from build123d import *

# Parameters (mm, degrees)
SKETCH2_W           = 54.8
SKETCH2_H           = 9.08
BOSS_EXTRUDE1_DEPTH = 6.49
SKETCH3_W           = 50
SKETCH3_H           = 6.43
CUT_EXTRUDE1_DEPTH  = 57.521498565
BOSS_EXTRUDE2_DEPTH = 6.49


with BuildPart() as part:
    # Sketch2 → Boss-Extrude1 (new body)
    with BuildSketch(Plane.XZ):
        with Locations((13.46, 33.97)):
            Rectangle(SKETCH2_W, SKETCH2_H)
    extrude(amount=BOSS_EXTRUDE1_DEPTH)

    # Sketch3 → Cut-Extrude1 (cut, through all)
    with BuildSketch(Plane(origin=(0, 0, 0), x_dir=(1, 0, 0), z_dir=(0, 1, 0))):
        with Locations((13.46, -32.645)):
            Rectangle(SKETCH3_W, SKETCH3_H)
    extrude(amount=-CUT_EXTRUDE1_DEPTH, mode=Mode.SUBTRACT)

    # Sketch4 → Boss-Extrude2 (add, through all)
    with BuildSketch(Plane(origin=(0, 0, 0), x_dir=(1, 0, 0), z_dir=(0, 1, 0))):
        with BuildLine():
            Line((38.46, -29.43), (37.86, -29.43))
            ThreePointArc((37.86, -29.43), (37.36, -30.68), (37.86, -31.93))
            Line((37.86, -31.93), (38.46, -31.93))
            Line((38.46, -31.93), (38.46, -29.43))
        make_face()
        with BuildLine():
            Line((-10.94, -31.93), (-11.54, -31.93))
            Line((-11.54, -31.93), (-11.54, -29.43))
            Line((-11.54, -29.43), (-10.94, -29.43))
            ThreePointArc((-10.94, -29.43), (-10.44, -30.68), (-10.94, -31.93))
        make_face()
    extrude(amount=-BOSS_EXTRUDE2_DEPTH)


solid = part.part
The model under review builds one solid part; all positions refer to its coordinate system, in mm. A direction names the side the tool comes from. Give positions to 0.01 mm unless a question says otherwise; leave off trailing zeros. Write each loop counter-clockwise with the first axis right and the second up, starting at its lowest first coordinate (ties: lowest second). Pieces come first, ordered by that corner, then holes. Notation, with made-up numbers: M 87.25,53 L 106.25,53 A17 cw 106.25,77 Z; hole C 33,44 d6. An arc over 180 degrees is marked long. One line per question, with ' | ' between items. Start each with the question number.
Item 1: For pin 1 (1.5 mm diameter, centred on x = -3.5, z = 34, fed in from -Y); pin 2 (1.9 mm diameter, centred on x = 18, y = -2, fed in from -Z), all flat-tipped, find the tip position at first contact; note any pin that passes through.
Item 2: Draft analysis for pull direction X (two halves, no side actions). For faces 3 (the flat face through (-13.94, -3, 34)), 4 (the flat face through (13, -6.49, 37)), 5 (the flat face through (38.46, -3, 34)), state which applies: released by +X, released by -X, zero draft, split by the parting line, or undercut.
Item 3: We need section B-B on y = -5.5. Write out the cut boundary in (x, z) (1 decimal), plus the area to 3 significant figures.
Item 4: We need section C-C on z = 31. Write out the cut boundary in (x, y).
Item 5: We need section A-A on z = 34.75. Write out the cut boundary in (x, y).
Item 6: Wall thickness on line 1 (X direction, y = -4.5, z = 32); line 2 (Z direction, x = 29.5, y = -5); line 3 (Z direction, x = -11, y = -5.25): over which ranges is each line inside the solid? List them lowest first. Write a range as from..to.
Item 7: For faces 1 (the flat face through (-12, -3, 29.43)), 2 (the flat face through (-11.54, -3, 34)), list the 3-axis set-ups (+Z, -Z, +X, -X, +Y, -Y) from which the entire face can be reached by the end or side of a thin tool; tool diameter is ignored.
Item 8: We need section D-D on x = 29. Write out the cut boundary in (y, z).
Results found:
1) pin 1: passes through | pin 2: stops at z = 35.86
2) face 3: released by -X | face 4: zero draft | face 5: undercut
3) outline: M -13.9,29.4 L -10.9,29.4 A1.8 ccw -10.9,31.9 L -11.5,31.9 L -11.5,35.9 L 38.5,35.9 L 38.5,31.9 L 37.9,31.9 A1.8 ccw 37.9,29.4 L 40.9,29.4 L 40.9,38.5 L -13.9,38.5 Z | area: 181 mm2
4) outline: M -13.94,-6.49 L -10.47,-6.49 L -10.47,0 L -13.94,0 Z; M 37.39,-6.49 L 40.86,-6.49 L 40.86,0 L 37.39,0 Z
5) outline: M -13.94,-6.49 L -11.54,-6.49 L -11.54,0 L -13.94,0 Z; M 38.46,-6.49 L 40.86,-6.49 L 40.86,0 L 38.46,0 Z
6) line 1: x = -13.94..-11.54, 38.46..40.86 | line 2: z = 35.86..38.51 | line 3: z = 29.43..31.93, 35.86..38.51
7) face 1: -Z, +X, -X, +Y, -Y | face 2: +Y, -Y
8) outline: M -6.49,35.86 L 0,35.86 L 0,38.51 L -6.49,38.51 Z
